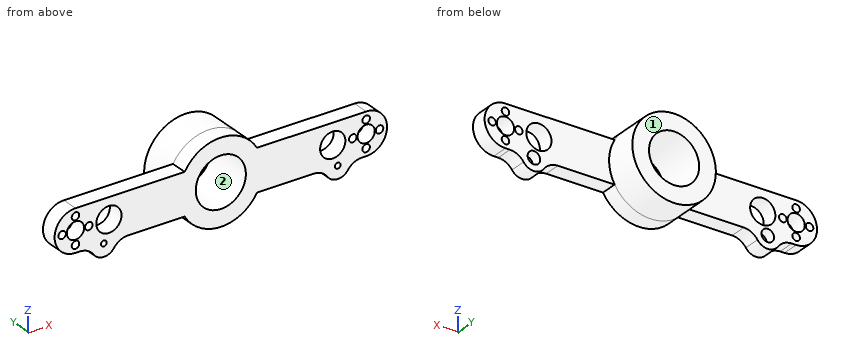
```python
from build123d import *

# Parameters (mm, degrees)
ESQUISSE1_R                                        = 5.15
ESQUISSE1_R_2                                      = 15
BOSS_EXTRU_1_DEPTH                                 = 10
DIAM_TRE_DU_PER_AGE_4_5_4_5_1_D                    = 4.5
R_P_TITION_CIRCULAIRE1_COUNT                       = 4
ESQUISSE4_R                                        = 7.55
ENL_V_MAT_EXTRU_1_DEPTH                            = 104.078853311
SYM_TRIE1_COPY_1_D                                 = 4.5
SYM_TRIE1_COPY_2_D                                 = 4.5
SYM_TRIE1_COPY_3_D                                 = 4.5
ESQUISSE7_R                                        = 25
ESQUISSE7_R_2                                      = 15
BOSS_EXTRU_3_DEPTH                                 = 20
BOSS_EXTRU_4_DEPTH                                 = 10
CHAMBRAGE_POUR_VIS_T_TE_RONDE_BOMB_E_M_D           = 3.4
CHAMBRAGE_POUR_VIS_T_TE_RONDE_BOMB_E_M_CBORE_D     = 7.5
CHAMBRAGE_POUR_VIS_T_TE_RONDE_BOMB_E_M_CBORE_DEPTH = 6.4
CONG_1_R                                           = 10


with BuildPart() as part:
    # Esquisse1 → Boss.-Extru.1 (new body)
    with BuildSketch(Plane(origin=(0, 0, 0), x_dir=(1, 0, 0), z_dir=(0, 1, 0))):
        with BuildLine():
            Line((87, -12.5), (21.650635095, -12.5))
            ThreePointArc((21.650635095, -12.5), (0, -25), (-21.650635095, -12.5))
            Line((-21.650635095, -12.5), (-87, -12.5))
            ThreePointArc((-87, -12.5), (-99.5, 0), (-87, 12.5))
            Line((-87, 12.5), (-21.650635095, 12.5))
            ThreePointArc((-21.650635095, 12.5), (0, 25), (21.650635095, 12.5))
            Line((21.650635095, 12.5), (87, 12.5))
            ThreePointArc((87, 12.5), (99.5, 0), (87, -12.5))
        make_face()
        with Locations(Location((-87, 0, 0), (0, 0, 270))):
            Circle(ESQUISSE1_R, mode=Mode.SUBTRACT)
        with Locations(Location((87, 0, 0), (0, 0, 270))):
            Circle(ESQUISSE1_R, mode=Mode.SUBTRACT)
        with Locations(Location((0, 0, 0), (0, 0, 270))):
            Circle(ESQUISSE1_R_2, mode=Mode.SUBTRACT)
    extrude(amount=BOSS_EXTRU_1_DEPTH)

    # Diamètre du perçage Ø4.5 (4.5)1 (through all)
    with Locations(Plane(origin=(0, 10, 0), x_dir=(1, 0, 0), z_dir=(0, 1, 0))):
        with Locations((-87, 8)):
            diam_tre_du_per_age_4_5_4_5_1 = Hole(DIAM_TRE_DU_PER_AGE_4_5_4_5_1_D / 2)

    # Répétition circulaire1: Diamètre du perçage Ø4.5 (4.5)1 ×4 about axis
    r_p_tition_circulaire1_axis = Axis((-87, 0, 0), (0, 1, 0))
    for i in range(1, R_P_TITION_CIRCULAIRE1_COUNT):
        add(diam_tre_du_per_age_4_5_4_5_1.rotate(r_p_tition_circulaire1_axis, i * 360 / R_P_TITION_CIRCULAIRE1_COUNT), mode=Mode.SUBTRACT)

    # Esquisse4 → Enlèv. mat.-Extru.1 (cut, through all)
    with BuildSketch(Plane(origin=(0, 10, 0), x_dir=(1, 0, 0), z_dir=(0, 1, 0))):
        with Locations(Location((-67, 0, 0), (0, 0, 270))):
            Circle(ESQUISSE4_R)
    enl_v_mat_extru_1 = extrude(amount=-ENL_V_MAT_EXTRU_1_DEPTH, mode=Mode.SUBTRACT)

    # Symétrie1: Diamètre du perçage Ø4.5 (4.5)1, Enlèv. mat.-Extru.1 across plane
    add(diam_tre_du_per_age_4_5_4_5_1.mirror(Plane(origin=(0, 0, 0), x_dir=(0, 0, 1), z_dir=(1, 0, 0))), mode=Mode.SUBTRACT)
    add(enl_v_mat_extru_1.mirror(Plane(origin=(0, 0, 0), x_dir=(0, 0, 1), z_dir=(1, 0, 0))), mode=Mode.SUBTRACT)

    # Symétrie1 copy 1 (through all)
    with Locations(Plane(origin=(87, 10, -87), x_dir=(0, 0, -1), z_dir=(0, 1, 0))):
        with Locations((-87, -8)):
            Hole(SYM_TRIE1_COPY_1_D / 2)

    # Symétrie1 copy 2 (through all)
    with Locations(Plane(origin=(174, 10, 0), x_dir=(1, 0, 0), z_dir=(0, 1, 0))):
        with Locations((-87, -8)):
            Hole(SYM_TRIE1_COPY_2_D / 2)

    # Symétrie1 copy 3 (through all)
    with Locations(Plane(origin=(87, 10, 87), x_dir=(0, 0, 1), z_dir=(0, 1, 0))):
        with Locations((-87, -8)):
            Hole(SYM_TRIE1_COPY_3_D / 2)

    # Esquisse7 → Boss.-Extru.3 (add)
    with BuildSketch(Plane(origin=(0, 10, 0), x_dir=(1, 0, 0), z_dir=(0, 1, 0))):
        with Locations(Location((0, 0, 0), (0, 0, 30))):
            Circle(ESQUISSE7_R)
        with Locations(Location((0, 0, 0), (0, 0, 270))):
            Circle(ESQUISSE7_R_2, mode=Mode.SUBTRACT)
    extrude(amount=BOSS_EXTRU_3_DEPTH)

    # Esquisse8 → Boss.-Extru.4 (add, through all)
    with BuildSketch(Plane(origin=(0, 10, 0), x_dir=(1, 0, 0), z_dir=(0, 1, 0))):
        with BuildLine():
            Line((62.5, 12.5), (77.5, 12.5))
            ThreePointArc((77.5, 12.5), (70, 20), (62.5, 12.5))
        make_face()
        with BuildLine():
            Line((-62.5, 12.5), (-77.5, 12.5))
            ThreePointArc((-77.5, 12.5), (-70, 20), (-62.5, 12.5))
        make_face()
    extrude(amount=-BOSS_EXTRU_4_DEPTH)

    # Chambrage pour vis à tête ronde bombée M31 (through all)
    with Locations(Plane(origin=(0, 10, 0), x_dir=(1, 0, 0), z_dir=(0, 1, 0))):
        with Locations((70, 12.5), (-70, 12.5)):
            CounterBoreHole(CHAMBRAGE_POUR_VIS_T_TE_RONDE_BOMB_E_M_D / 2, CHAMBRAGE_POUR_VIS_T_TE_RONDE_BOMB_E_M_CBORE_D / 2, CHAMBRAGE_POUR_VIS_T_TE_RONDE_BOMB_E_M_CBORE_DEPTH)

    # Congé1
    cong_1_edges = [part.edges().sort_by_distance(p)[0] for p in [
        (62.5, 5, -12.5),
        (77.5, 5, -12.5),
        (-77.5, 5, -12.5),
        (-62.5, 5, -12.5),
    ]]
    fillet(cong_1_edges, radius=CONG_1_R)


solid = part.part
```
Model file for the job. Use its own axes, mm. Face numbers are marked on the shaded views. Give positions to 0.01 mm unless a question says otherwise; leave off trailing zeros. Order: outer loops, then holes, each group sorted by start corner. A loop starts at its lowest first (then second) coordinate and runs counter-clockwise, first axis right, second up.
1) Saw through at A-A, the plane x = 0. Write the cut outline in (y, z).
2) Wall check: probe 1 along Z at (x, y) = (70, 8); probe 2 along Y at (x, z) = (52.5, 4.5); probe 3 along Z at (x, y) = (70, 2.65). Give the ranges that are in metal, low to high.
3) Saw through at C-C, the plane z = 18. Write the cut outline in (x, y), then the cut area to 3 significant figures.
4) Saw through at B-B, the plane y = 8.25. Count the separate pieces of the cut face and the enclosed holes in it, then the cut area to 3 significant figures.
5) Mould opens along X. For the marked faces 1 and 2 say: +X half, -X half, draft (parallel to the pull), parting line (faces both ways), or undercut.
6) Saw through at D-D, the plane x = 95. Write the cut outline in (y, z), then the cut area to 3 significant figures.
7) Pin check, flat tips, straight feed: pin 1 (3 mm diameter, centred on x = -33, y = 5.5, fed in from -Z); pin 2 (12 mm diameter, centred on y = 10.5, z = -10.5, fed in from +X); pin 3 (3 mm diameter, centred on x = -58.5, y = 5.5, fed in from +Z). Stop position of each tip, or through.
Computed:
1. outline: (0, -25) - (30, -25) - (30, -15) - (0, -15) - close; (0, 15) - (30, 15) - (30, 25) - (0, 25) - close
2. probe 1: z = -20 to -16.25, -8.75 to -6.93, 6.93 to 12.5
2. probe 2: y = 0 to 10
2. probe 3: z = -20 to -14.2, -10.8 to -6.93, 6.93 to 12.5
3. outline: (-17.35, 0) - (17.35, 0) - (17.35, 30) - (-17.35, 30) - close
3. area: 1,040 mm2
4. separate pieces: 1
4. enclosed holes: 15
4. area: 4,360 mm2
5. face 1: draft
5. face 2: undercut
6. outline: (0, -9.6) - (10, -9.6) - (10, -2.25) - (0, -2.25) - close; (0, 2.25) - (10, 2.25) - (10, 9.6) - (0, 9.6) - close
6. area: 147 mm2
7. pin 1: stops at z = -12.5
7. pin 2: stops at x = 98.65
7. pin 3: stops at z = 12.5
